```python
from build123d import *

# Parameters (mm, degrees)
F0_W     = 70.9361852596
F0_H     = 59.7819101843
F0_R     = 6.35
F1_DEPTH = 25.4
F2_DEPTH = 6.35
F3_DEPTH = 25.4
F4_DEPTH = 25.4


with BuildPart() as f1:
    # F0 (on Front) → F1 (new body)
    with BuildSketch(Plane.XZ):
        with Locations((1.6176216304, -4.4821556658)):
            Rectangle(F0_W, F0_H)
        with Locations((-18.6856686208, 0)):
            Circle(F0_R, mode=Mode.SUBTRACT)
        with Locations((24.4943313792, 0)):
            Circle(F0_R, mode=Mode.SUBTRACT)
        with Locations((-18.6856686208, 0)):
            Circle(F0_R)
        with Locations((24.4943313792, 0)):
            Circle(F0_R)
    extrude(amount=-F1_DEPTH)

    # F0 (on Front) → F2 (join)
    with BuildSketch(Plane.XZ):
        with Locations((-18.6856686208, 0)):
            Circle(F0_R)
        with Locations((24.4943313792, 0)):
            Circle(F0_R)
    extrude(amount=F2_DEPTH)

    # F3 (add): a face of the model
    f3_faces = [f1.faces().sort_by_distance(p)[0] for p in [
        (37.0857142603, 12.7, -4.4821556658),
    ]]
    extrude(f3_faces, amount=F3_DEPTH)

    # F4 (add): a face of the model
    f4_faces = [f1.faces().sort_by_distance(p)[0] for p in [
        (-33.8504709994, 12.7, -4.4821556658),
    ]]
    extrude(f4_faces, amount=F4_DEPTH)


solid = f1.part
```
Input: part model. Units: mm. Frame: model coordinates. Give positions to 0.01 mm unless a question says otherwise; leave off trailing zeros. Loops run counter-clockwise (first coordinate to the right, second up) from the corner with the lowest first, then second, coordinate; pieces in that order, holes last. Notation, with made-up numbers: (41, -18) -> (67, -18) arc R23 ccw to (67, 18) -> close; hole circle Ø9 at (-0.75, 72.25). An arc over 180 degrees is marked (long way). Use a Markdown table: item, result.
Q1. Section query A-A, the plane z = 0. Return the cut outline in (x, y).
Entries:
| item | result |
|---|---|
| outline | (-59.25, 0) -> (-25.04, 0) -> (-25.04, -6.35) -> (-12.34, -6.35) -> (-12.34, 0) -> (18.14, 0) -> (18.14, -6.35) -> (30.84, -6.35) -> (30.84, 0) -> (62.49, 0) -> (62.49, 25.4) -> (-59.25, 25.4) -> close |
Q2. Section query D-D, the plane z = -15. Return the cut outline in (x, y), plus the area to 3 significant figures.
Entries:
| item | result |
|---|---|
| outline | (-59.25, 0) -> (62.49, 0) -> (62.49, 25.4) -> (-59.25, 25.4) -> close |
| area | 3,090 mm² |
Q3. Section query B-B, the plane x = 22. Return the cut outline in (y, z).
Entries:
| item | result |
|---|---|
| outline | (-6.35, -5.84) -> (0, -5.84) -> (0, -34.37) -> (25.4, -34.37) -> (25.4, 25.41) -> (0, 25.41) -> (0, 5.84) -> (-6.35, 5.84) -> close |
Q4. Section query C-C, the plane x = -8. Return the cut outline in (y, z), plus the area to 3 significant figures.
Entries:
| item | result |
|---|---|
| outline | (0, -34.37) -> (25.4, -34.37) -> (25.4, 25.41) -> (0, 25.41) -> close |
| area | 1,520 mm² |
Q5. Ray query, probe 1 along Y at (x, z) = (-1.5, -18); probe 2 along X at (y, z) = (-1, -5.5). Return the intervals inside material, ascending. Write a range as from..to.
Entries:
| item | result |
|---|---|
| probe 1 | y = 0..25.4 |
| probe 2 | x = -21.86..-15.51, 21.32..27.67 |
Q6. Pull-direction query (X, two-part tool) for faces 1 (the flat face through (24, -6.35, 0)), 2 (the cylindrical face through (-23.725, -3.131, -3.864)), 3 (the cylindrical face through (18.15, -3.13, 0.28)), 4 (the flat face through (62.486, 13, -5)); classes: pulls with the +X half, pulls with the -X half, needs draft (parallel to the pull), parting line crosses it, or undercut.
Entries:
| item | result |
|---|---|
| face 1 | needs draft |
| face 2 | undercut |
| face 3 | undercut |
| face 4 | pulls with the +X half |
